```python
from build123d import *

# Parameters (mm, degrees)
SKETCH1_W               = 381
SKETCH1_H               = 381
SKETCH1_R               = 4.064
SKETCH1_R_2             = 2.54
SKETCH1_R_3             = 6.223
SKETCH1_R_4             = 2.25
SKETCH1_R_5             = 2.5796875
SKETCH1_R_6             = 1.5875
BOSS_EXTRUDE1_DEPTH     = 6.35
F_3_8_24_TAPPED_HOLE2_D = 8.4328


with BuildPart() as part:
    # Sketch1 → Boss-Extrude1 (new body)
    with BuildSketch(Plane.XY):
        with Locations((0, 190.5)):
            Rectangle(SKETCH1_W, SKETCH1_H)
        with Locations((76.2, 273.05)):
            Circle(SKETCH1_R, mode=Mode.SUBTRACT)
        with Locations((44.45, 241.3)):
            Circle(SKETCH1_R_2, mode=Mode.SUBTRACT)
        with Locations((88.9, 95.25)):
            Circle(SKETCH1_R_3, mode=Mode.SUBTRACT)
        with Locations(Location((-165.1, 25.4, 0), (0, 0, 180))):
            Circle(SKETCH1_R_2, mode=Mode.SUBTRACT)
        with Locations((100.948737342, 297.798737342)):
            Circle(SKETCH1_R_4, mode=Mode.SUBTRACT)
        with Locations((158.75, 190.5)):
            Circle(SKETCH1_R_2, mode=Mode.SUBTRACT)
        with Locations((51.451262658, 297.798737342)):
            Circle(SKETCH1_R_4, mode=Mode.SUBTRACT)
        with Locations((165.1, 25.4)):
            Circle(SKETCH1_R_2, mode=Mode.SUBTRACT)
        with Locations(Location((-88.9, 95.25, 0), (0, 0, 180))):
            Circle(SKETCH1_R_3, mode=Mode.SUBTRACT)
        with Locations((28.575, 206.115)):
            Circle(SKETCH1_R_5, mode=Mode.SUBTRACT)
        with Locations(Location((-146.05, 190.5, 0), (0, 0, 180))):
            Circle(SKETCH1_R_2, mode=Mode.SUBTRACT)
        with Locations((-25.4, 301.365)):
            Circle(SKETCH1_R_5, mode=Mode.SUBTRACT)
        with Locations((25.4, 301.365)):
            Circle(SKETCH1_R_5, mode=Mode.SUBTRACT)
        with Locations(Location((-44.45, 241.3, 0), (0, 0, 180))):
            Circle(SKETCH1_R_2, mode=Mode.SUBTRACT)
        with Locations(Location((-76.2, 273.05, 0), (0, 0, 180))):
            Circle(SKETCH1_R, mode=Mode.SUBTRACT)
        with Locations((-28.575, 206.115)):
            Circle(SKETCH1_R_5, mode=Mode.SUBTRACT)
        with Locations((-95.25, 316.23)):
            Circle(SKETCH1_R_6, mode=Mode.SUBTRACT)
        with Locations((100.948737342, 248.301262658)):
            Circle(SKETCH1_R_4, mode=Mode.SUBTRACT)
    extrude(amount=BOSS_EXTRUDE1_DEPTH)

    # 3/8-24 Tapped Hole2 (through all)
    with Locations(Plane.XY.offset(6.35)):
        with Locations((-146.05, 254)):
            Hole(F_3_8_24_TAPPED_HOLE2_D / 2)


solid = part.part
```
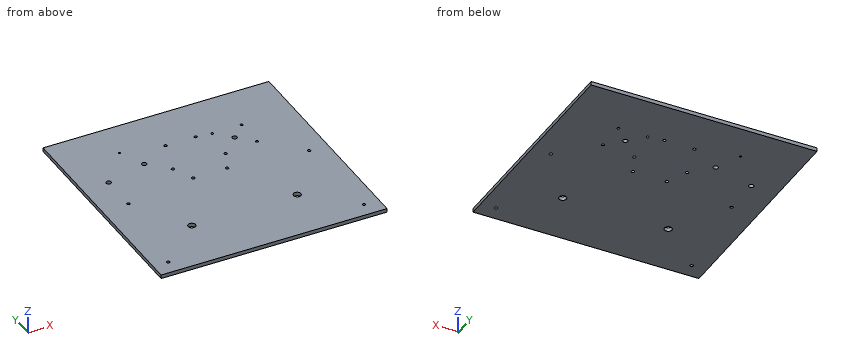
Check sheet for the modelled part. Datum: model origin and axes. Units: mm. Round coordinates to 2 decimals unless told otherwise and drop trailing zeros. Loops run counter-clockwise (first coordinate to the right, second up) from the corner with the lowest first, then second, coordinate; pieces in that order, holes last. Notation, with made-up numbers: (73.25, -29.5) - (118.25, -29.5) arc R18 ccw to (118.25, -23.5) - close; hole circle Ø6 at (65, -11.75). An arc over 180 degrees is marked (long way). Write item = value, one per line. Start each with the question number.
Q1. Depth check by flat-ended pin: P1, Ø7.5, axis at x = -88.9, y = 95.25, coming from the +Z side. Enter the tip coordinate at first touch or a pass-through.
Q2. Thickness scan on L1, parallel to X at y = 273.05, z = 3.25; L2, parallel to X at y = 190.5, z = 2; L3, parallel to Y at x = 100.5, z = 4.25. Record the ranges inside material, lowest first.
Q3. Section check A-A (x = -88.9). Record the boundary of the cut face in (y, z), plus the area to 3 significant figures.
Derived:
q1.P1 = through
q2.L1 = -190.5 to -80.26, -72.14 to 72.14, 80.26 to 190.5
q2.L2 = -190.5 to -148.59, -143.51 to 156.21, 161.29 to 190.5
q2.L3 = 0 to 246.1, 250.51 to 295.59, 300 to 381
q3.outline = (0, 0) - (89.03, 0) - (89.03, 6.35) - (0, 6.35) - close; (101.47, 0) - (381, 0) - (381, 6.35) - (101.47, 6.35) - close
q3.area = 2,340 mm^2
